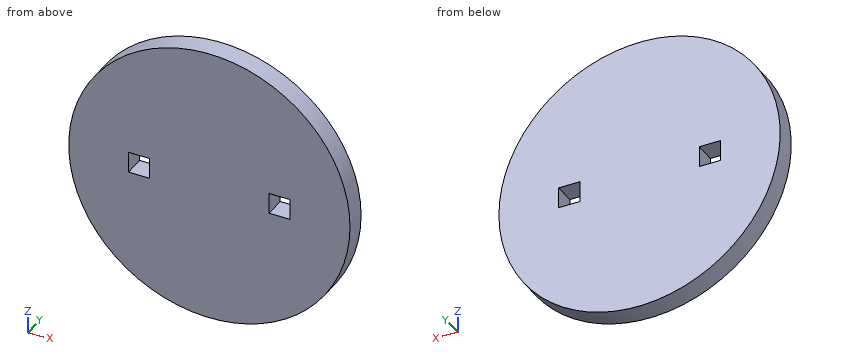
```python
from build123d import *

# Parameters (mm, degrees)
CROQUIS1_R              = 40
CROQUIS1_W              = 6
CROQUIS1_H              = 6
SALIENTE_EXTRUIR1_DEPTH = 6


with BuildPart() as part:
    # Croquis1 → Saliente-Extruir1 (new body)
    with BuildSketch(Plane(origin=(0, 0, 0), x_dir=(1, 0, 0), z_dir=(0, 1, 0))):
        Circle(CROQUIS1_R)
        with Locations((-20, 0)):
            Rectangle(CROQUIS1_W, CROQUIS1_H, mode=Mode.SUBTRACT)
        with Locations((20, 0)):
            Rectangle(CROQUIS1_W, CROQUIS1_H, mode=Mode.SUBTRACT)
    extrude(amount=SALIENTE_EXTRUIR1_DEPTH)


solid = part.part
```
For this review, take the finished solid that the model builds, in its own axes (mm). Round coordinates to 2 decimals unless told otherwise and drop trailing zeros. Loops run counter-clockwise (first coordinate to the right, second up) from the corner with the lowest first, then second, coordinate; pieces in that order, holes last.
(1) We need section C-C (z = 21). Give the boundary of the cut face in (x, y).
Returned:
outline: (-34.04, 0) - (34.04, 0) - (34.04, 6) - (-34.04, 6) - close
(2) Wall thickness on line 1 along X through (y, z) = (3.15, 0); line 2 along Z through (x, y) = (-21.5, 1.7); line 3 along Z through (x, y) = (18, 1.7): over which ranges is each line inside the solid? List them lowest first.
Returned:
line 1: x = -40 to -23, -17 to 17, 23 to 40
line 2: z = -33.73 to -3, 3 to 33.73
line 3: z = -35.72 to -3, 3 to 35.72
(3) We need section D-D (x = -11.5). Give the boundary of the cut face in (y, z).
Returned:
outline: (0, -38.31) - (6, -38.31) - (6, 38.31) - (0, 38.31) - close
(4) We need section A-A (z = 0). Give the boundary of the cut face in (x, y).
Returned:
outline: (-40, 0) - (-23, 0) - (-23, 6) - (-40, 6) - close; (-17, 0) - (17, 0) - (17, 6) - (-17, 6) - close; (23, 0) - (40, 0) - (40, 6) - (23, 6) - close
(5) We need section B-B (y = 2.6). Give the boundary of the cut face in (x, z).
Returned:
outline: circle Ø80 at (0, 0); hole (-23, -3) - (-17, -3) - (-17, 3) - (-23, 3) - close; hole (17, -3) - (23, -3) - (23, 3) - (17, 3) - close
(6) Clearance check with flat-ended pins moving along their axes: P1, Ø1, axis at y = 3.5, z = 19.5, coming from the +X side; P2, Ø1, axis at x = -3.5, y = 2, coming from the -Z side; P3, Ø3, axis at x = 19, y = 3.5, coming from the +Z side. State where each tip first meets the part, or that it passes through.
Returned:
P1: stops at x = 35.2
P2: stops at z = -39.89
P3: stops at z = 35.97
